Model file for the job. Use its own axes, mm. A direction names the side the tool comes from. Coordinates: 2 decimals unless noted, no trailing zeros. Order: outer loops, then holes, each group sorted by start corner. A loop starts at its lowest first (then second) coordinate and runs counter-clockwise, first axis right, second up.
from build123d import *

# Parameters (mm, degrees)
F1_DEPTH = 25.4


with BuildPart() as f1:
    # F0 (on Front) → F1 (new body)
    with BuildSketch(Plane.XZ):
        with BuildLine():
            Line((76.2, 266.7), (76.2, 292.1))
            Line((76.2, 292.1), (-76.2, 292.1))
            Line((-76.2, 292.1), (-76.2, -292.1))
            Line((-76.2, -292.1), (76.2, -292.1))
            Line((76.2, -292.1), (76.2, -212.725))
            Line((76.2, -212.725), (36.5125, -228.6))
            ThreePointArc((36.5125, -228.6), (25.4, -239.7125), (14.2875, -228.6))
            Line((14.2875, -228.6), (14.2875, -222.788529))
            ThreePointArc((14.2875, -222.788529), (16.198103, -216.558541), (21.272921, -212.470832))
            Line((21.272921, -212.470832), (76.2, -190.5))
            Line((76.2, -190.5), (76.2, -161.925))
            Line((76.2, -161.925), (36.5125, -177.8))
            ThreePointArc((36.5125, -177.8), (25.4, -188.9125), (14.2875, -177.8))
            Line((14.2875, -177.8), (14.2875, -171.988529))
            ThreePointArc((14.2875, -171.988529), (16.198103, -165.758541), (21.272921, -161.670832))
            Line((21.272921, -161.670832), (76.2, -139.7))
            Line((76.2, -139.7), (76.2, -111.125))
            Line((76.2, -111.125), (36.5125, -127))
            ThreePointArc((36.5125, -127), (25.4, -138.1125), (14.2875, -127))
            Line((14.2875, -127), (14.2875, -121.188529))
            ThreePointArc((14.2875, -121.188529), (16.198103, -114.958541), (21.272921, -110.870832))
            Line((21.272921, -110.870832), (76.2, -88.9))
            Line((76.2, -88.9), (76.2, -60.325))
            Line((76.2, -60.325), (36.5125, -76.2))
            ThreePointArc((36.5125, -76.2), (25.4, -87.3125), (14.2875, -76.2))
            Line((14.2875, -76.2), (14.2875, -70.388529))
            ThreePointArc((14.2875, -70.388529), (16.198103, -64.158541), (21.272921, -60.070832))
            Line((21.272921, -60.070832), (76.2, -38.1))
            Line((76.2, -38.1), (76.2, -9.525))
            Line((76.2, -9.525), (36.5125, -25.4))
            ThreePointArc((36.5125, -25.4), (25.4, -36.5125), (14.2875, -25.4))
            Line((14.2875, -25.4), (14.2875, -19.588529))
            ThreePointArc((14.2875, -19.588529), (16.198103, -13.358541), (21.272921, -9.270832))
            Line((21.272921, -9.270832), (76.2, 12.7))
            Line((76.2, 12.7), (76.2, 41.275))
            Line((76.2, 41.275), (36.5125, 25.4))
            ThreePointArc((36.5125, 25.4), (25.4, 14.2875), (14.2875, 25.4))
            Line((14.2875, 25.4), (14.2875, 31.211471))
            ThreePointArc((14.2875, 31.211471), (16.198103, 37.441459), (21.272921, 41.529168))
            Line((21.272921, 41.529168), (76.2, 63.5))
            Line((76.2, 63.5), (76.2, 92.075))
            Line((76.2, 92.075), (36.5125, 76.2))
            ThreePointArc((36.5125, 76.2), (25.4, 65.0875), (14.2875, 76.2))
            Line((14.2875, 76.2), (14.2875, 82.011471))
            ThreePointArc((14.2875, 82.011471), (16.198103, 88.241459), (21.272921, 92.329168))
            Line((21.272921, 92.329168), (76.2, 114.3))
            Line((76.2, 114.3), (76.2, 142.875))
            Line((76.2, 142.875), (36.5125, 127))
            ThreePointArc((36.5125, 127), (25.4, 115.8875), (14.2875, 127))
            Line((14.2875, 127), (14.2875, 132.811471))
            ThreePointArc((14.2875, 132.811471), (16.198103, 139.041459), (21.272921, 143.129168))
            Line((21.272921, 143.129168), (76.2, 165.1))
            Line((76.2, 165.1), (76.2, 193.675))
            Line((76.2, 193.675), (36.5125, 177.8))
            ThreePointArc((36.5125, 177.8), (25.4, 166.6875), (14.2875, 177.8))
            Line((14.2875, 177.8), (14.2875, 183.611471))
            ThreePointArc((14.2875, 183.611471), (16.198103, 189.841459), (21.272921, 193.929168))
            Line((21.272921, 193.929168), (76.2, 215.9))
            Line((76.2, 215.9), (76.2, 244.475))
            Line((76.2, 244.475), (36.5125, 228.6))
            ThreePointArc((36.5125, 228.6), (25.4, 217.4875), (14.2875, 228.6))
            Line((14.2875, 228.6), (14.2875, 234.411471))
            ThreePointArc((14.2875, 234.411471), (16.198103, 240.641459), (21.272921, 244.729168))
            Line((21.272921, 244.729168), (76.2, 266.7))
        make_face()
    extrude(amount=F1_DEPTH)


solid = f1.part
Q1. Mould opens along Z. For faces 4 (the face through (16.147, -12.522, 189.765)), 5 (the face through (76.2, -13, -253)) say: pulls with the +Z half, pulls with the -Z half, needs draft (parallel to the pull), parting line crosses it, or undercut.
Established:
face 4: undercut
face 5: needs draft
Q2. Cut at B-B, the plane x = 57. Count the separate pieces of the cut face and the enclosed holes in it, plus the area to 3 significant figures.
Established:
separate pieces: 11
enclosed holes: 0
area: 9,190 mm2
Q3. Cut at C-C, the plane z = -43. List the corners of the cut face in (x, y).
Established:
outline: (-76.2, -25.4) - (63.95, -25.4) - (63.95, 0) - (-76.2, 0) - close
Q4. Cut at A-A, the plane z = 57.5. List the corners of the cut face in (x, y), plus the area to 3 significant figures.
Established:
outline: (-76.2, -25.4) - (61.2, -25.4) - (61.2, 0) - (-76.2, 0) - close
area: 3,490 mm2
Q5. Which spindle directions (+Z, -Z, +X, -X, +Y, -Y) get a long thin tool onto all of the face, cutting with end or side? Do faces 1 (the face through (16.147, -12.522, -115.035)), 2 (the face through (48.35, -12.52, 153.96)), 3 (the face through (76.2, -13, 279)). Say none if no direction does.
Established:
face 1: +Y, -Y
face 2: +X, +Y, -Y
face 3: +Z, -Z, +X, +Y, -Y
Q6. Probe line 1 (X direction, y = -21.5, z = 221.5); line 2 (X direction, y = -24, z = 114); line 3 (X direction, y = -17.75, z = -198.5). List the from-to ranges inside material, lowest first.
Established:
line 1: x = -76.2 to 16.85, 33.95 to 76.2
line 2: x = -76.2 to 75.45
line 3: x = -76.2 to 56.2
